Geometry: see drawing. Coordinates: mm, zero at the bounding-box minimum. A direction names the side the tool comes from. Round coordinates to 2 decimals unless told otherwise and drop trailing zeros. Loops run counter-clockwise (first coordinate to the right, second up) from the corner with the lowest first, then second, coordinate; pieces in that order, holes last. Notation, with made-up numbers: (59.5, -12.5) - (84.5, -12.5) arc R28 cw to (84.5, 26.5) - close; hole circle Ø2 at (-6.5, -6). An arc over 180 degrees is marked (long way). Write item = value, one per line. Start each with the question number.
Item 1: Draft query along Z for the marked faces 3, 4, 5 and 6. Return one class per face: pulls with the +Z half, pulls with the -Z half, needs draft (parallel to the pull), parting line crosses it, or undercut.
Item 2: Section A-A (x = 22.8). Return loops of the section in (y, z).
Item 3: Section C-C (z = 5.85). Return loops of the section in (x, y).
Item 4: Line query: line 1 (Z direction, x = 22.8, y = 14.5); line 2 (X direction, y = 5.5, z = 7); line 3 (Z direction, x = 5.8, y = 2.75). Output: solid intervals per line, ascending. Write a range as from..to.
Item 5: Access query for the marked faces 1 and 2. Directions: +Z, -Z, +X, -X, +Y, -Y. A direction counts if a zero-diameter tool reaches every point of the face in a straight line with its end or side. Return the directions, or none.
Item 6: First-contact query: pin 1 (3 mm diameter, centred on x = 5.8, z = 5.85, fed in from -Y); pin 2 (1 mm diameter, centred on x = 7.5, z = 6.5, fed in from -Y); pin 3 (3 mm diameter, centred on x = 17.5, y = 4, fed in from +Z). Flat tips, straight axial feed; report the tip coordinate or a pass-through.
Item 7: Section D-D (z = 3.75). Return loops of the section in (x, y).
Item 8: Section B-B (y = 12.75). Return loops of the section in (x, z).
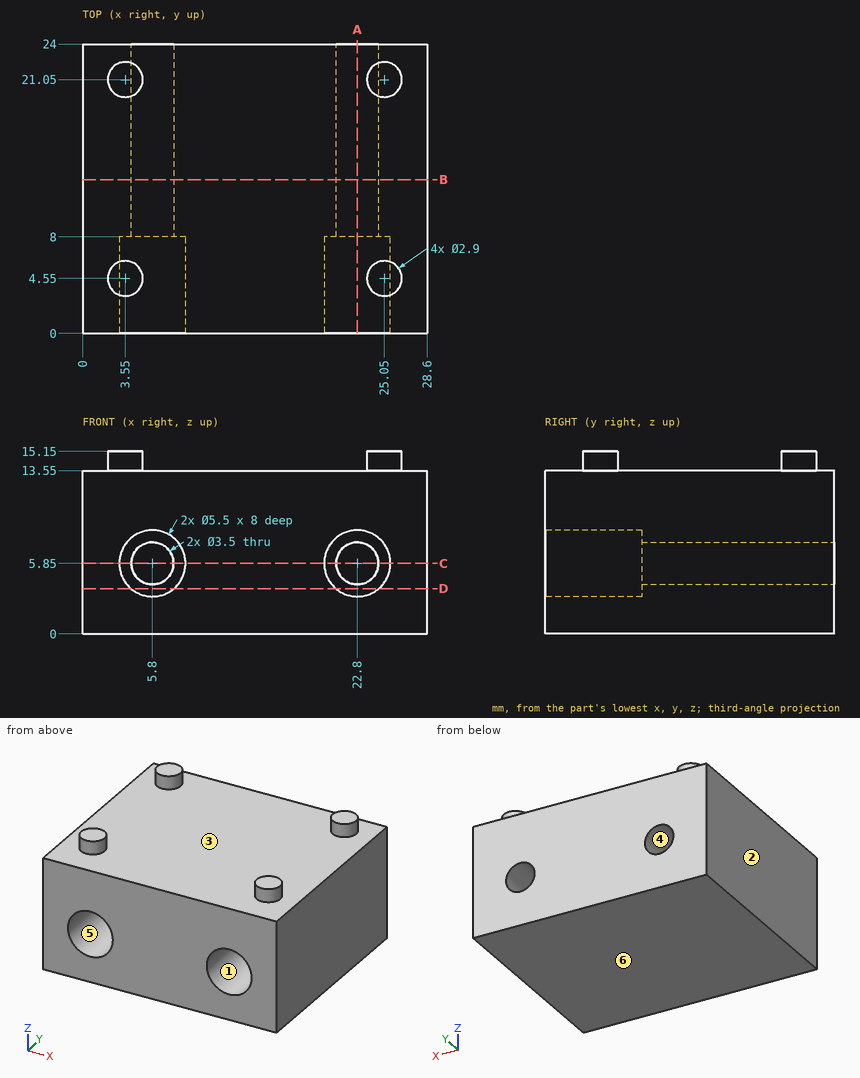
Taken from the geometry:
q1.face_3 = pulls with the +Z half
q1.face_4 = undercut
q1.face_5 = undercut
q1.face_6 = pulls with the -Z half
q2.outline = (0, 0) - (24, 0) - (24, 4.1) - (8, 4.1) - (8, 3.1) - (0, 3.1) - close; (0, 8.6) - (8, 8.6) - (8, 7.6) - (24, 7.6) - (24, 13.55) - (0, 13.55) - close
q3.outline = (0, 0) - (3.05, 0) - (3.05, 8) - (4.05, 8) - (4.05, 24) - (0, 24) - close; (7.55, 8) - (8.55, 8) - (8.55, 0) - (20.05, 0) - (20.05, 8) - (21.05, 8) - (21.05, 24) - (7.55, 24) - close; (24.55, 8) - (25.55, 8) - (25.55, 0) - (28.6, 0) - (28.6, 24) - (24.55, 24) - close
q4.line_1 = 0..4.1, 7.6..13.55
q4.line_2 = 0..3.3, 8.3..20.3, 25.3..28.6
q4.line_3 = 0..3.1, 8.6..13.55
q5.face_1 = -Y
q5.face_2 = +Z, -Z, -X, +Y, -Y
q6.pin_1 = through
q6.pin_2 = 8
q6.pin_3 = 13.55
q7.outline = (0, 0) - (4.02, 0) - (4.02, 8) - (7.58, 8) - (7.58, 0) - (21.02, 0) - (21.02, 8) - (24.58, 8) - (24.58, 0) - (28.6, 0) - (28.6, 24) - (0, 24) - close
q8.outline = (0, 0) - (28.6, 0) - (28.6, 13.55) - (0, 13.55) - close; hole circle Ø3.5 at (5.8, 5.85); hole circle Ø3.5 at (22.8, 5.85)
